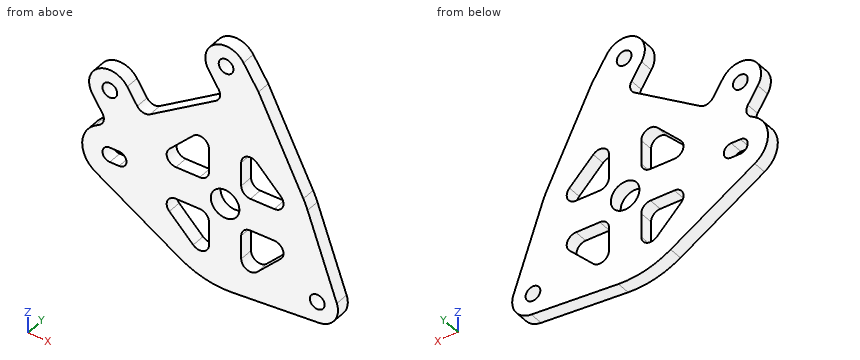
from build123d import *

# Parameters (mm, degrees)
SKETCH_1_R      = 3.1
SKETCH_1_R_2    = 1.6
EXTRUDE_1_DEPTH = 3
FILLET_1_R      = 2


with BuildPart() as part:
    # 草图1 → 凸台-拉伸1 (new body)
    with BuildSketch(Plane(origin=(0, 0, 0), x_dir=(1, 0, 0), z_dir=(0, 1, 0))):
        with BuildLine():
            Line((-82.094284463, 13.64505302), (-75.759172636, 31.494880978))
            ThreePointArc((-75.759172636, 31.494880978), (-76.227003727, 35.452447578), (-79.653832636, 37.486665594))
            Line((-79.653832636, 37.486665594), (-98.538404465, 38.943699177))
            ThreePointArc((-98.538404465, 38.943699177), (-104.422619767, 38.478106894), (-109.88, 36.229158943))
            Line((-109.88, 36.229158943), (-128.12, 25.124997561))
            ThreePointArc((-128.12, 25.124997561), (-130.999516523, 20.076167551), (-128.249103426, 14.955862123))
            Line((-128.249103426, 14.955862123), (-125.533999982, 13.206970217))
            Line((-125.533999982, 13.206970217), (-128.783103408, 8.16283234))
            ThreePointArc((-128.783103408, 8.16283234), (-127.43682757, 1.942901362), (-121.216896592, 3.289177201))
            Line((-121.216896592, 3.289177201), (-117.967793166, 8.333315078))
            Line((-117.967793166, 8.333315078), (-100.313310595, -3.038546913))
            Line((-100.313310595, -3.038546913), (-103.562414021, -8.08268479))
            ThreePointArc((-103.562414021, -8.08268479), (-102.216138182, -14.302615768), (-95.996207205, -12.956339929))
            Line((-95.996207205, -12.956339929), (-92.747103778, -7.912202052))
            Line((-92.747103778, -7.912202052), (-83.017679727, 11.479389802))
            ThreePointArc((-83.017679727, 11.479389802), (-82.522406202, 12.547905325), (-82.094284463, 13.64505302))
        make_face()
        Polygon((-96.5, 16.5), (-84.5, 16.5), (-96.5, 4.5), align=None, mode=Mode.SUBTRACT)
        Polygon((-103.5, 16.5), (-103.5, 4.5), (-115.5, 16.5), align=None, mode=Mode.SUBTRACT)
        Polygon((-103.5, 23.5), (-115.5, 23.5), (-103.5, 35.5), align=None, mode=Mode.SUBTRACT)
        Polygon((-96.5, 23.5), (-96.5, 35.5), (-84.5, 23.5), align=None, mode=Mode.SUBTRACT)
        with Locations(Location((-100, 20, 0), (0, 0, 270))):
            Circle(SKETCH_1_R, mode=Mode.SUBTRACT)
        with Locations(Location((-80, 33, 0), (0, 0, 270))):
            Circle(SKETCH_1_R_2, mode=Mode.SUBTRACT)
        with BuildLine():
            Line((-125, 21.6), (-123, 21.6))
            ThreePointArc((-123, 21.6), (-121.4, 20), (-123, 18.4))
            Line((-123, 18.4), (-125, 18.4))
            ThreePointArc((-125, 18.4), (-126.6, 20), (-125, 21.6))
        make_face(mode=Mode.SUBTRACT)
        with Locations(Location((-99.779310613, -10.51951236, 0), (0, 0, 270))):
            Circle(SKETCH_1_R_2, mode=Mode.SUBTRACT)
        with Locations(Location((-125, 5.726004771, 0), (0, 0, 270))):
            Circle(SKETCH_1_R_2, mode=Mode.SUBTRACT)
    extrude(amount=EXTRUDE_1_DEPTH)

    # 圆角1
    fillet_1_edges = [part.edges().sort_by_distance(p)[0] for p in [
        (-96.5, 1.5, -16.5),
        (-96.5, 1.5, -4.5),
        (-84.5, 1.5, -16.5),
        (-103.5, 1.5, -4.5),
        (-103.5, 1.5, -16.5),
        (-115.5, 1.5, -16.5),
        (-115.5, 1.5, -23.5),
        (-103.5, 1.5, -23.5),
        (-103.5, 1.5, -35.5),
        (-96.5, 1.5, -35.5),
        (-96.5, 1.5, -23.5),
        (-84.5, 1.5, -23.5),
        (-100.313310595, 1.5, 3.038546913),
        (-117.967793166, 1.5, -8.333315078),
        (-125.533999982, 1.5, -13.206970217),
    ]]
    fillet(fillet_1_edges, radius=FILLET_1_R)


solid = part.part
Design review of the part built by this model. Coordinates are the model's own, in mm. Give positions to 0.01 mm unless a question says otherwise; leave off trailing zeros. Write each loop counter-clockwise with the first axis right and the second up, starting at its lowest first coordinate (ties: lowest second). Pieces come first, ordered by that corner, then holes. Notation, with made-up numbers: M 79,-2.75 L 126,-2.75 A31 cw 126,34.25 Z; hole C 49,43 d8. An arc over 180 degrees is marked long. Return JSON: item names as keys, results as strings. Group by question number.
Item 1: Take a section at C-C (z = 0). Give the boundary of the cut face in (x, y), plus the area to 3 significant figures.
Item 2: Take a section at A-A (z = -20). Give the boundary of the cut face in (x, y).
Item 3: Clearance check with flat-ended pins moving along their axes: pin 1 Ø1.5 at (y, z) = (2, -11.5) entering from -X; pin 2 Ø0.9 at (x, y) = (-107, 1) entering from +Z; pin 3 Ø3 at (x, z) = (-99.78, 10.52) entering from -Y; pin 4 Ø1.5 at (x, z) = (-93, 9.5) entering from -Y. State where each tip first meets the part, or that it passes through.
Item 4: Wall thickness on line 1 along X through (y, z) = (1.15, -20); line 2 along Z through (x, y) = (-124, 2.1) (3 decimals); line 3 along Z through (x, y) = (-98.5, 1.85): over which ranges is each line inside the solid? List them lowest first.
Item 5: Take a section at B-B (y = 2.1). Count the separate pieces of the cut face and the enclosed holes in it, plus the area to 3 significant figures.
Return value:
{
 "1": {"outline": "M -105.03,0 L -88.78,0 L -88.78,3 L -105.03,3 Z", "area": "48.8 mm2"},
 "2": {"outline": "M -131,0 L -126.6,0 L -126.6,3 L -131,3 Z; M -121.4,0 L -103.1,0 L -103.1,3 L -121.4,3 Z; M -96.9,0 L -79.84,0 L -79.84,3 L -96.9,3 Z"},
 "3": {"pin 1": "stops at x = -127.12", "pin 2": "stops at z = -0.98", "pin 3": "passes through", "pin 4": "stops at y = 0"},
 "4": {"line 1": "x = -131 to -126.6, -121.4 to -103.1, -96.9 to -79.84", "line 2": "z = -27.633 to -21.6, -18.4 to -6.975, -4.477 to -1.339", "line 3": "z = -38.94 to -22.71, -17.29 to 9.56, 11.48 to 14.83"},
 "5": {"separate pieces": "1", "enclosed holes": "9", "area": "1,440 mm2"}
}
